The model under review builds one solid part; all positions refer to its coordinate system, in mm. A direction names the side the tool comes from. Coordinates: 2 decimals unless noted, no trailing zeros. Loops run counter-clockwise (first coordinate to the right, second up) from the corner with the lowest first, then second, coordinate; pieces in that order, holes last. Notation, with made-up numbers: (51.25, 65) - (61.25, 65) arc R37 ccw to (61.25, 101) - close; hole circle Ø7 at (-25.75, 72.5). An arc over 180 degrees is marked (long way). Use a Markdown table: item, result. Add a question column.
1) To check wall thickness, follow L1, parallel to X at y = -41, z = 0.75; L2, parallel to X at y = -66, z = 2.25; L3, parallel to X at y = -31, z = 6.5. State the ranges of each line that lie inside material, in increasing order. Write a range as [from, to].
2) Clearance check with flat-ended pins moving along their axes: pin 1 (3 mm diameter, centred on y = -30.5, z = 5.5, fed in from -X); pin 2 (8 mm diameter, centred on x = 11.5, y = 5.5, fed in from +Z); pin 3 (1.6 mm diameter, centred on x = 13.5, z = 8, fed in from +Y). State where each tip first meets the part, or that it passes through.
3) Add section A-A, the plane y = -37. Give the boundary of the cut face in (x, z), and give its area (3 significant figures).
4) Add section B-B, the plane x = 17. Give the boundary of the cut face in (y, z), and give its area (3 significant figures).
5) For faces 5 (the cylindrical face through (63.698, -68.425, 1.22)), 6 (the flat face through (41.141, -43, 3)), 7 (the flat face through (10, -107.098, 3)), 8 (the flat face through (-23, -2.098, 5)), list the 3-axis set-ups (+Z, -Z, +X, -X, +Y, -Y) from which the entire face can be reached by the end or side of a thin tool; tool diameter is ignored.
6) The part is to be moulded in two halves that separate along X. For faces 1 (the cylindrical face through (-45.495, -67.672, 1.22)), 2 (the flat face through (-38, 22, 4.5)), 3 (the flat face through (-52.359, -48, 1)), 4 (the flat face through (-8.859, -41, 1)), say which applies: pulls with the +X half, pulls with the -X half, needs draft (parallel to the pull), parting line crosses it, or undercut.
```python
from build123d import *

# Parameters (mm, degrees)
ESBO_O1_W                                    = 125
ESBO_O1_H                                    = 140
RESSALTO_EXTRUS_O1_DEPTH                     = 2.5
RESSALTO_EXTRUS_O2_DEPTH                     = 6
ESBO_O3_W                                    = 1.52
ESBO_O3_H                                    = 105
CORTE_EXTRUS_O1_DEPTH                        = 2
ESBO_O4_W                                    = 1.52
ESBO_O4_H                                    = 105
CORTE_EXTRUS_O2_DEPTH                        = 2
ESBO_O5_W                                    = 66
ESBO_O5_H                                    = 1.52
CORTE_EXTRUS_O3_DEPTH                        = 2
FILETE1_R                                    = 2
FILETE2_R                                    = 2
FILETE3_R                                    = 2
ESBO_O6_W                                    = 12
ESBO_O6_H                                    = 130
CORTE_EXTRUS_O4_DEPTH                        = 138.929522592
FILETE4_R                                    = 2
FILETE5_R                                    = 2
ESBO_O7_W                                    = 19.009766083
ESBO_O7_H                                    = 4
ESBO_O7_W_2                                  = 19
ESBO_O7_W_3                                  = 29.5
RESSALTO_EXTRUS_O3_DEPTH                     = 2
ESBO_O8_W                                    = 123
ESBO_O8_H                                    = 1.1
CORTE_EXTRUS_O5_DEPTH                        = 2
FILETE6_R                                    = 2
FUROS_GUIA_COM_3_0MM1_D                      = 3
FUROS_GUIA_COM_3_0MM1_CSINK_D                = 3.05
FUROS_GUIA_COM_3_0MM1_CSINK_ANGLE            = 90
REBAIXO_PARA_PARAFUSO_COM_CABE_A_PAN_2_COUNT = 2
REBAIXO_PARA_PARAFUSO_COM_CABE_A_PAN_2_PITCH = 101


with BuildPart() as part:
    # Esboço1 → Ressalto-extrusão1 (new body)
    with BuildSketch(Plane.XY):
        with Locations((10.140586838, -47.097815293)):
            Rectangle(ESBO_O1_W, ESBO_O1_H)
    extrude(amount=RESSALTO_EXTRUS_O1_DEPTH)

    # Esboço2 → Ressalto-extrusão2 (add)
    with BuildSketch(Plane.XY.offset(2.5)):
        Polygon((-24.859413162, -2.097815293), (-20.859413162, -2.097815293), (-20.859413162, -107.097815293), (41.140586838, -107.097815293), (41.140586838, -2.097815293), (45.140586838, -2.097815293), (45.140586838, -107.097815293), (45.140586838, -111.097815293), (-24.859413162, -111.097815293), (-24.859413162, -107.097815293), align=None)
    extrude(amount=RESSALTO_EXTRUS_O2_DEPTH)

    # Esboço3 → Corte-extrusão1 (cut)
    with BuildSketch(Plane.ZY.offset(-41.140586838)):
        with Locations((6.26, -54.597815293)):
            Rectangle(ESBO_O3_W, ESBO_O3_H)
    extrude(amount=-CORTE_EXTRUS_O1_DEPTH, mode=Mode.SUBTRACT)

    # Esboço4 → Corte-extrusão2 (cut)
    with BuildSketch(Plane(origin=(-20.859413162, 0, 0), x_dir=(0, 0, -1), z_dir=(1, 0, 0))):
        with Locations((-6.26, -54.597815293)):
            Rectangle(ESBO_O4_W, ESBO_O4_H)
    extrude(amount=-CORTE_EXTRUS_O2_DEPTH, mode=Mode.SUBTRACT)

    # Esboço5 → Corte-extrusão3 (cut)
    with BuildSketch(Plane(origin=(0, -107.097815293, 0), x_dir=(1, 0, 0), z_dir=(0, 1, 0))):
        with Locations((10.140586838, -6.26)):
            Rectangle(ESBO_O5_W, ESBO_O5_H)
    extrude(amount=-CORTE_EXTRUS_O3_DEPTH, mode=Mode.SUBTRACT)

    # Filete1
    filete1_edges = [part.edges().sort_by_distance(p)[0] for p in [
        (41.140586838, -107.097815293, 7.76),
        (-20.859413162, -107.097815293, 7.76),
        (41.140586838, -107.097815293, 4),
        (-20.859413162, -107.097815293, 4),
    ]]
    fillet(filete1_edges, radius=FILETE1_R)

    # Filete2
    filete2_edges = [part.edges().sort_by_distance(p)[0] for p in [
        (-24.859413162, -111.097815293, 5.5),
        (45.140586838, -111.097815293, 5.5),
    ]]
    fillet(filete2_edges, radius=FILETE2_R)

    # Filete3
    filete3_edges = [part.edges().sort_by_distance(p)[0] for p in [
        (10.140586838, -111.097815293, 2.5),
        (-24.273626724, -110.512028855, 2.5),
        (44.5548004, -110.512028855, 2.5),
        (-24.859413162, -55.597815293, 2.5),
        (45.140586838, -55.597815293, 2.5),
    ]]
    fillet(filete3_edges, radius=FILETE3_R)

    # Esboço6 → Corte-extrusão4 (cut, through all)
    with BuildSketch(Plane.XY.offset(2.5)):
        with Locations((-14.859413162, -42.097815293)):
            Rectangle(ESBO_O6_W, ESBO_O6_H)
        with Locations((35.140586838, -42.097815293)):
            Rectangle(ESBO_O6_W, ESBO_O6_H)
    extrude(amount=-CORTE_EXTRUS_O4_DEPTH, mode=Mode.SUBTRACT)

    # Filete4
    filete4_edges = [part.edges().sort_by_distance(p)[0] for p in [
        (-20.859413162, 22.902184707, 1.25),
        (-8.859413162, 22.902184707, 1.25),
        (41.140586838, 22.902184707, 1.25),
        (29.140586838, 22.902184707, 1.25),
    ]]
    fillet(filete4_edges, radius=FILETE4_R)

    # Filete5
    filete5_edges = [part.edges().sort_by_distance(p)[0] for p in [
        (-20.859413162, -107.097815293, 1.25),
        (-8.859413162, -107.097815293, 1.25),
        (41.140586838, -107.097815293, 1.25),
        (29.140586838, -107.097815293, 1.25),
    ]]
    fillet(filete5_edges, radius=FILETE5_R)

    # Esboço7 → Ressalto-extrusão3 (add)
    with BuildSketch(Plane.XY.offset(2.5)):
        with Locations((0.635703797, 20.902184707)):
            Rectangle(ESBO_O7_W, ESBO_O7_H)
        with Locations((19.640586838, 20.902184707)):
            Rectangle(ESBO_O7_W_2, ESBO_O7_H)
        with Locations((-37.609413162, 20.902184707)):
            Rectangle(ESBO_O7_W_3, ESBO_O7_H)
        with Locations((57.890586838, 20.902184707)):
            Rectangle(ESBO_O7_W_3, ESBO_O7_H)
    extrude(amount=RESSALTO_EXTRUS_O3_DEPTH)

    # Esboço8 → Corte-extrusão5 (cut)
    with BuildSketch(Plane.XY.offset(4.5)):
        with Locations((11.140586838, 20.902184707)):
            Rectangle(ESBO_O8_W, ESBO_O8_H)
    extrude(amount=-CORTE_EXTRUS_O5_DEPTH, mode=Mode.SUBTRACT)

    # Filete6
    # the kernel refuses this fillet: 2 mm, written as the material it adds along each edge
    with BuildSketch(Plane(origin=(29.140586838, 18.902184707, 2.5), x_dir=(0, 0, 1), z_dir=(-1, 0, 0))) as filete6_piece_1:
        with BuildLine():
            CenterArc((FILETE6_R, -FILETE6_R), FILETE6_R, 90, 90)
            Line((0, -FILETE6_R), (0, 0))
            Line((0, 0), (FILETE6_R, 0))
        make_face()
    extrude(amount=38)
    with BuildSketch(Plane(origin=(-52.359413162, 18.902184707, 2.5), x_dir=(0, 0, 1), z_dir=(1, 0, 0)), Plane(origin=(43.140586838, 18.902184707, 2.5), x_dir=(0, 0, 1), z_dir=(1, 0, 0))) as filete6_piece_2:
        with BuildLine():
            CenterArc((FILETE6_R, FILETE6_R), FILETE6_R, 180, 90)
            Line((0, FILETE6_R), (0, 0))
            Line((0, 0), (FILETE6_R, 0))
        make_face()
    extrude(amount=29.5)
    # the kernel refuses this fillet: 2 mm, written as the material it takes off along each edge
    with BuildSketch(Plane(origin=(29.140586838, 22.902184707, -2.307221131), x_dir=(-1, 0, 0), z_dir=(0, 0, 1))) as filete6_2_piece_1:
        with BuildLine():
            CenterArc((1.922888452, 2), FILETE6_R, 195.962014163, 74.037985837)
            Line((0, 1.45), (0, 0))
            Line((0, 0), (1.922888452, 0))
        make_face()
    extrude(amount=11.614442262, mode=Mode.SUBTRACT)
    with BuildSketch(Plane(origin=(-8.869179245, 22.902184707, -2.307221131), x_dir=(1, 0, 0), z_dir=(0, 0, 1))) as filete6_2_piece_2:
        with BuildLine():
            CenterArc((1.922888452, -2), FILETE6_R, 90, 74.037985837)
            Line((0, -1.45), (0, 0))
            Line((0, 0), (1.922888452, 0))
        make_face()
    extrude(amount=11.614442262, mode=Mode.SUBTRACT)

    # Furos-guia com Ø3.0mm1 (through all)
    with Locations(Plane.XY.offset(2.5)):
        with Locations((-44.109413162, -27.097815293), (-44.109413162, -67.097815293), (64.390586838, -27.094030717), (64.390586838, -67.094030814)):
            CounterSinkHole(FUROS_GUIA_COM_3_0MM1_D / 2, FUROS_GUIA_COM_3_0MM1_CSINK_D / 2, counter_sink_angle=FUROS_GUIA_COM_3_0MM1_CSINK_ANGLE)

    # Esboço14 → Rebaixo para parafuso com cabeça panela de M31 (revolve, cut)
    with BuildSketch(Plane(origin=(-40.359413162, -108.297815293, 0), x_dir=(0, 1, 0), z_dir=(1, 0, 0))):
        Polygon((0, 0), (0, 8.5), (1.7, 8.5), (1.7, 2.4), (3.5, 2.4), (3.5, 0.025), (3.525, 0), align=None)
    rebaixo_para_parafuso_com_cabe_a_panela = revolve(axis=Axis((-40.359413162, -108.297815293, -6.35), (0, 0, 1)), mode=Mode.SUBTRACT)

    # Rebaixo para parafuso com cabe_a pan 2: Rebaixo para parafuso com cabeça panela de M31 ×2
    with Locations(*[(i * REBAIXO_PARA_PARAFUSO_COM_CABE_A_PAN_2_PITCH, 0, 0) for i in range(1, REBAIXO_PARA_PARAFUSO_COM_CABE_A_PAN_2_COUNT)]):
        add(rebaixo_para_parafuso_com_cabe_a_panela, mode=Mode.SUBTRACT)


solid = part.part
```
From the geometry:
| question | item | result |
|---|---|---|
| 1 | L1 | x = [-52.36, -20.86], [-8.86, 29.14], [41.14, 72.64] |
| 1 | L2 | x = [-52.36, -45.13], [-43.09, -20.86], [-8.86, 29.14], [41.14, 63.36], [65.42, 72.64] |
| 1 | L3 | x = [-24.86, -22.86], [43.14, 45.14] |
| 2 | pin 1 | stops at x = -24.92 |
| 2 | pin 2 | stops at z = 2.5 |
| 2 | pin 3 | stops at y = -107.1 |
| 3 | outline | (-52.36, 0) - (-20.86, 0) - (-20.86, 5.5) - (-22.86, 5.5) - (-22.86, 7.02) - (-20.86, 7.02) - (-20.86, 8.5) - (-24.86, 8.5) - (-24.86, 4.5) arc R2 cw to (-26.86, 2.5) - (-52.36, 2.5) - close; (-8.86, 0) - (29.14, 0) - (29.14, 2.5) - (-8.86, 2.5) - close; (41.14, 0) - (72.64, 0) - (72.64, 2.5) - (47.14, 2.5) arc R2 cw to (45.14, 4.5) - (45.14, 8.5) - (41.14, 8.5) - (41.14, 7.02) - (43.14, 7.02) - (43.14, 5.5) - (41.14, 5.5) - close |
| 3 | area | 296 mm^2 |
| 4 | outline | (-117.1, 0) - (22.9, 0) - (22.9, 4.5) - (21.45, 4.5) - (21.45, 2.5) - (20.35, 2.5) - (20.35, 4.5) - (18.9, 4.5) arc R2 cw to (16.9, 2.5) - (-107.1, 2.5) - (-107.1, 5.5) - (-109.1, 5.5) - (-109.1, 7.02) - (-107.1, 7.02) - (-107.1, 8.5) - (-111.1, 8.5) - (-111.1, 4.5) arc R2 cw to (-113.1, 2.5) - (-117.1, 2.5) - close |
| 4 | area | 378 mm^2 |
| 5 | face 5 | +Z, -Z |
| 5 | face 6 | +Z, -Z, +Y |
| 5 | face 7 | +Z |
| 5 | face 8 | +Z, +X, -X |
| 6 | face 1 | undercut |
| 6 | face 2 | needs draft |
| 6 | face 3 | pulls with the -X half |
| 6 | face 4 | undercut |
